from build123d import *

# Parameters (mm, degrees)
SKETCH4_W           = 40
SKETCH4_H           = 40
BOSS_EXTRUDE3_DEPTH = 5
SKETCH1_W           = 36
SKETCH1_H           = 36
SKETCH1_W_2         = 26
SKETCH1_H_2         = 26
BOSS_EXTRUDE4_DEPTH = 35
SKETCH9_W           = 50
SKETCH9_H           = 50
SKETCH9_W_2         = 26
SKETCH9_H_2         = 26
BOSS_EXTRUDE6_DEPTH = 5
SKETCH10_R          = 1.75
CUT_EXTRUDE2_DEPTH  = 10
CUT_EXTRUDE3_DEPTH  = 10


with BuildPart() as part:
    # Sketch4 → Boss-Extrude3 (new body)
    with BuildSketch(Plane(origin=(0, 0, 0), x_dir=(1, 0, 0), z_dir=(0, 1, 0))):
        Rectangle(SKETCH4_W, SKETCH4_H)
        Polygon((-2.5, -8.525), (-2.5, -13), (-13, -13), (-13, -2.5), (-8.400446417, -2.5), (-4.921911045, -8.525), align=None, mode=Mode.SUBTRACT)
        Polygon((7.534421013, 0), (3.767210506, 6.525), (-3.767210506, 6.525), (-7.534421013, 0), (-3.767210506, -6.525), (3.767210506, -6.525), align=None, mode=Mode.SUBTRACT)
        Polygon((13, 13), (2.5, 13), (2.5, 8.525), (4.921911045, 8.525), (8.400446417, 2.5), (13, 2.5), align=None, mode=Mode.SUBTRACT)
        Polygon((13, -13), (2.5, -13), (2.5, -8.525), (4.921911045, -8.525), (8.400446417, -2.5), (13, -2.5), align=None, mode=Mode.SUBTRACT)
        Polygon((-13, 13), (-13, 2.5), (-8.400446417, 2.5), (-4.921911045, 8.525), (-2.5, 8.525), (-2.5, 13), align=None, mode=Mode.SUBTRACT)
    extrude(amount=BOSS_EXTRUDE3_DEPTH)

    # Sketch1 → Boss-Extrude4 (add)
    with BuildSketch(Plane(origin=(0, 0, 0), x_dir=(1, 0, 0), z_dir=(0, 1, 0))):
        Rectangle(SKETCH1_W, SKETCH1_H)
        Rectangle(SKETCH1_W_2, SKETCH1_H_2, mode=Mode.SUBTRACT)
    extrude(amount=BOSS_EXTRUDE4_DEPTH)

    # Sketch9 → Boss-Extrude6 (add)
    with BuildSketch(Plane(origin=(0, 30, 0), x_dir=(1, 0, 0), z_dir=(0, 1, 0))):
        Rectangle(SKETCH9_W, SKETCH9_H)
        Rectangle(SKETCH9_W_2, SKETCH9_H_2, mode=Mode.SUBTRACT)
    extrude(amount=BOSS_EXTRUDE6_DEPTH)

    # Sketch10 → Cut-Extrude2 (cut)
    with BuildSketch(Plane(origin=(0, 25, 0), x_dir=(1, 0, 0), z_dir=(0, 1, 0))):
        with Locations((-21.25, 21.25)):
            Circle(SKETCH10_R)
        with Locations((21.25, 21.25)):
            Circle(SKETCH10_R)
        with Locations((21.25, -21.25)):
            Circle(SKETCH10_R)
        with Locations((-21.25, -21.25)):
            Circle(SKETCH10_R)
    extrude(amount=CUT_EXTRUDE2_DEPTH, mode=Mode.SUBTRACT)

    # Sketch11 → Cut-Extrude3 (cut)
    with BuildSketch(Plane(origin=(0, 25, 0), x_dir=(1, 0, 0), z_dir=(0, 1, 0))):
        Polygon((11, 18), (-11, 18), (-18, 25), (18, 25), align=None)
        Polygon((18, 11), (18, -11), (25, -18), (25, 18), align=None)
        Polygon((11, -18), (-11, -18), (-18, -25), (18, -25), align=None)
        Polygon((-18, 11), (-18, -11), (-25, -18), (-25, 18), align=None)
    extrude(amount=CUT_EXTRUDE3_DEPTH, mode=Mode.SUBTRACT)


solid = part.part
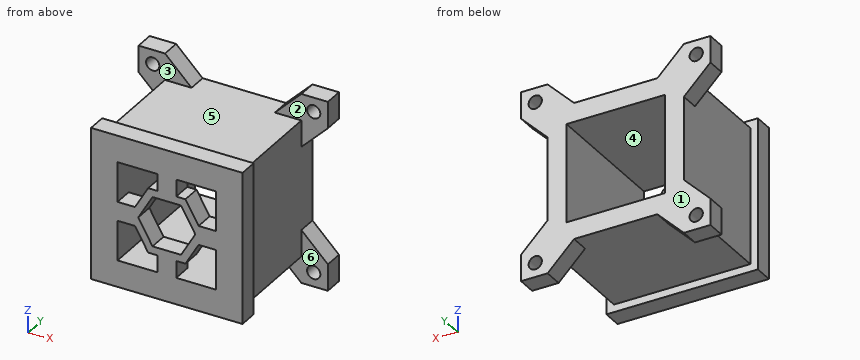
Read the model definition and answer for the solid it produces. Units are mm, in the model's axes. Face numbers are marked on the shaded views. A direction names the side the tool comes from. Coordinates: 2 decimals unless noted, no trailing zeros. Order: outer loops, then holes, each group sorted by start corner. A loop starts at its lowest first (then second) coordinate and runs counter-clockwise, first axis right, second up. Notation, with made-up numbers: M 34,-33.75 L 71,-33.75 A26 ccw 71,-13.75 Z; hole C -33.5,45.5 d3. An arc over 180 degrees is marked long. Put each result on its own line as item: value. Start each with the question number.
Item 1: Consider probe 1 along X at (y, z) = (3, -9.5); probe 2 along Z at (x, y) = (7.5, 32); probe 3 along Z at (x, y) = (-21.25, 31.1). Determine where each line is inside the solid, lowest interval first. Write a range as [from, to].
Item 2: Section D-D, the plane y = 20.5 is taken. Determine the outline of the cut face in (x, z).
Item 3: The mould has two halves that part along Z. Classify the marked faces 4, 5 and 6: +Z half, -Z half, draft (parallel to the pull), parting line (faces both ways), or undercut.
Item 4: Section B-B, the plane y = 33 is taken. Determine the outline of the cut face in (x, z), plus the area to 3 significant figures.
Item 5: Section A-A, the plane z = -21.25 is taken. Determine the outline of the cut face in (x, y).
Item 6: For the marked faces 1, 2 and 3, determine the directions among +Z, -Z, +X, -X, +Y, -Y from which every point of the face is accessible in a straight line to the end or side of a thin tool.
Item 7: Section C-C, the plane x = -21.25 is taken. Determine the outline of the cut face in (y, z), plus the area to 3 significant figures.
Item 8: Given pin 1 Ø1.5 at (x, y) = (2.5, 3.5) entering from +Z; pin 2 Ø2 at (x, z) = (-9.5, 14.5) entering from -Y; pin 3 Ø3 at (x, y) = (-10, 16) entering from -Z; pin 4 Ø2.5 at (x, y) = (4, 2) entering from -Z, each flat-ended and moving along its own axis, determine where each tip first touches the part or whether it passes through.
Computed:
1. probe 1: x = [-20, -13], [-2.5, 2.5], [13, 20]
1. probe 2: z = [-18, -13], [13, 18]
1. probe 3: z = [-25, -23], [-19.5, -14.25], [14.25, 19.5], [23, 25]
2. outline: M -18,-18 L 18,-18 L 18,18 L -18,18 Z; hole M -13,-13 L 13,-13 L 13,13 L -13,13 Z
3. face 4: undercut
3. face 5: +Z half
3. face 6: draft
4. outline: M -25,-25 L -18,-25 L -11,-18 L 11,-18 L 18,-25 L 25,-25 L 25,-18 L 18,-11 L 18,11 L 25,18 L 25,25 L 18,25 L 11,18 L -11,18 L -18,25 L -25,25 L -25,18 L -18,11 L -18,-11 L -25,-18 Z; hole C -21.25,-21.25 d3.5; hole C -21.25,21.25 d3.5; hole M -13,-13 L 13,-13 L 13,13 L -13,13 Z; hole C 21.25,-21.25 d3.5; hole C 21.25,21.25 d3.5
4. area: 974 mm2
5. outline: M -25,30 L -23,30 L -23,35 L -25,35 Z; M -19.5,30 L -14.25,30 L -14.25,35 L -19.5,35 Z; M 14.25,30 L 19.5,30 L 19.5,35 L 14.25,35 Z; M 23,30 L 25,30 L 25,35 L 23,35 Z
6. face 1: +Z, -Z, +X, -X, +Y
6. face 2: +Z, +X
6. face 3: +Z, -X
7. outline: M 30,-25 L 35,-25 L 35,-23 L 30,-23 Z; M 30,-19.5 L 35,-19.5 L 35,-14.25 L 30,-14.25 Z; M 30,14.25 L 35,14.25 L 35,19.5 L 30,19.5 Z; M 30,23 L 35,23 L 35,25 L 30,25 Z
7. area: 72.5 mm2
8. pin 1: stops at z = 20
8. pin 2: stops at y = 0
8. pin 3: stops at z = -18
8. pin 4: stops at z = -20
